```python
from build123d import *

# Parameters (mm, degrees)
SKETCH1_R               = 1.25
BOSS_EXTRUDE1_DEPTH     = 2
BOSS_EXTRUDE2_DEPTH     = 7.5
SKETCH3_R               = 1.25
CUT_EXTRUDE1_DEPTH      = 2
CUT_EXTRUDE1_DEPTH_BACK = 4


with BuildPart() as part:
    # Sketch1 → Boss-Extrude1 (new body)
    with BuildSketch(Plane.XY):
        Polygon((1952.176808721, 1466.884115951), (1957.176808721, 1466.884115951), (1957.176808721, 1462.884115951), (1958.426808721, 1462.884115951), (1958.426808721, 1458.884115951), (1957.176808721, 1458.884115951), (1957.176808721, 1454.884115951), (1952.176808721, 1454.884115951), (1952.176808721, 1458.884115951), (1950.926808721, 1458.884115951), (1950.926808721, 1462.884115951), (1952.176808721, 1462.884115951), align=None)
        with Locations((1954.676808721, 1460.884115951)):
            Circle(SKETCH1_R, mode=Mode.SUBTRACT)
    extrude(amount=BOSS_EXTRUDE1_DEPTH)

    # Sketch2 → Boss-Extrude2 (add)
    with BuildSketch(Plane.ZY.offset(-1950.926808721)):
        with BuildLine():
            Line((2, 1458.884115951), (2, 1459.884115951))
            ThreePointArc((2, 1459.884115951), (2.292893219, 1459.17700917), (3, 1458.884115951))
            Line((3, 1458.884115951), (2, 1458.884115951))
        make_face()
        with BuildLine():
            Line((0, 1458.884115951), (-1, 1458.884115951))
            ThreePointArc((-1, 1458.884115951), (-0.292893219, 1459.17700917), (0, 1459.884115951))
            Line((0, 1459.884115951), (0, 1458.884115951))
        make_face()
    extrude(amount=-BOSS_EXTRUDE2_DEPTH)

    # Sketch3 → Cut-Extrude1 (cut, two sides)
    with BuildSketch(Plane.XY.offset(2)) as cut_extrude1_sk:
        with Locations((1954.676808721, 1460.884115951)):
            Circle(SKETCH3_R)
    extrude(amount=CUT_EXTRUDE1_DEPTH, mode=Mode.SUBTRACT)
    extrude(cut_extrude1_sk.sketch, amount=-CUT_EXTRUDE1_DEPTH_BACK, mode=Mode.SUBTRACT)


solid = part.part
```
Input: part model. Units: mm. Frame: model coordinates. A direction names the side the tool comes from. Give positions to 0.01 mm unless a question says otherwise; leave off trailing zeros. Loops run counter-clockwise (first coordinate to the right, second up) from the corner with the lowest first, then second, coordinate; pieces in that order, holes last. Notation, with made-up numbers: (-8.5, 68.25) -> (22.5, 68.25) arc R18 ccw to (22.5, 72.25) -> close; hole circle Ø10 at (1, 7). An arc over 180 degrees is marked (long way). Use a Markdown table: item, result.
Q1. Ray query, probe 1 along Z at (x, y) = (1955.75, 1465.75); probe 2 along X at (y, z) = (1460.25, 1.3); probe 3 along Y at (x, z) = (1955.75, 1.35). Return the intervals inside material, ascending. Write a range as from..to.
Entries:
| item | result |
|---|---|
| probe 1 | z = 0..2 |
| probe 2 | x = 1950.93..1953.6, 1955.75..1958.43 |
| probe 3 | y = 1454.88..1460.24, 1461.53..1466.88 |
Q2. Pull-direction query (X, two-part tool) for faces 4 (the flat face through (1952.177, 1457, 1)), 5 (the flat face through (1958, 1462.884, 1)), 6 (the cylindrical face through (1953.685, 1460.124, 0.986)); classes: pulls with the +X half, pulls with the -X half, needs draft (parallel to the pull), parting line crosses it, or undercut.
Entries:
| item | result |
|---|---|
| face 4 | pulls with the -X half |
| face 5 | needs draft |
| face 6 | undercut |
Q3. Section query B-B, the plane x = 1956.25. Return the cut outline in (y, z).
Entries:
| item | result |
|---|---|
| outline | (1454.88, 0) -> (1458.88, 0) -> (1458.88, -1) arc R1 cw to (1459.88, 0) -> (1466.88, 0) -> (1466.88, 2) -> (1459.88, 2) arc R1 cw to (1458.88, 3) -> (1458.88, 2) -> (1454.88, 2) -> close |
Q4. Section query D-D, the plane z = 0.7. Return the cut outline in (x, y).
Entries:
| item | result |
|---|---|
| outline | (1950.93, 1458.88) -> (1952.18, 1458.88) -> (1952.18, 1454.88) -> (1957.18, 1454.88) -> (1957.18, 1458.88) -> (1958.43, 1458.88) -> (1958.43, 1462.88) -> (1957.18, 1462.88) -> (1957.18, 1466.88) -> (1952.18, 1466.88) -> (1952.18, 1462.88) -> (1950.93, 1462.88) -> close; hole circle Ø2.5 at (1954.68, 1460.88) |
Q5. Access query for faces 1 (the flat face through (1957.177, 1465, 1)), 2 (the flat face through (1952, 1462.884, 1)), 3 (the flat face through (1955, 1457, 0)). Directions: +Z, -Z, +X, -X, +Y, -Y. A direction counts if a zero-diameter tool reaches every point of the face in a straight line with its end or side. Return the directions, or none.
Entries:
| item | result |
|---|---|
| face 1 | +Z, -Z, +X, +Y |
| face 2 | +Z, -Z, -X, +Y |
| face 3 | -Z, +X, -X, -Y |
Q6. Section query C-C, the plane y = 1461.25. Return the cut outline in (x, z).
Entries:
| item | result |
|---|---|
| outline | (1950.93, 0) -> (1953.48, 0) -> (1953.48, 2) -> (1950.93, 2) -> close; (1955.87, 0) -> (1958.43, 0) -> (1958.43, 2) -> (1955.87, 2) -> close |
Q7. Section query A-A, the plane x = 1954.5. Return the cut outline in (y, z).
Entries:
| item | result |
|---|---|
| outline | (1454.88, 0) -> (1458.88, 0) -> (1458.88, -1) arc R1 cw to (1459.65, -0.03) -> (1459.65, 2.03) arc R1 cw to (1458.88, 3) -> (1458.88, 2) -> (1454.88, 2) -> close; (1462.12, 0) -> (1466.88, 0) -> (1466.88, 2) -> (1462.12, 2) -> close |
Q8. First-contact query: P1, Ø3, axis at x = 1952.5, y = 1465, coming from the -Z side; P2, Ø1.2, axis at x = 1953.5, y = 1457, coming from the +Z side; P3, Ø0.6, axis at y = 1457.5, z = 0.5, coming from the -X side. Flat tips, straight axial feed; report the tip coordinate or a pass-through.
Entries:
| item | result |
|---|---|
| P1 | stops at z = 0 |
| P2 | stops at z = 2 |
| P3 | stops at x = 1952.18 |
